Source: CAD feature listing. Evaluate the final solid. Frame: model axes, mm. A direction names the side the tool comes from. Give positions to 0.01 mm unless a question says otherwise; leave off trailing zeros. Write each loop counter-clockwise with the first axis right and the second up, starting at its lowest first coordinate (ties: lowest second). Pieces come first, ordered by that corner, then holes. Notation, with made-up numbers: (40, 62) -> (89, 62) arc R30 ccw to (89, 93) -> close; hole circle Ø5 at (-15.5, -2.5). An arc over 180 degrees is marked (long way). Write item = value, one per line.
from build123d import *

# Parameters (mm, degrees)
BOSS_EXTRUDE1_DEPTH     = 10
SKETCH3_W               = 5
SKETCH3_H               = 10
BOSS_EXTRUDE2_DEPTH     = 10
SKETCH5_R               = 2.5
CUT_EXTRUDE1_DEPTH      = 20
MIRROR2_COPY_1_SKETCH_W = 5
MIRROR2_COPY_1_SKETCH_H = 10
MIRROR2_COPY_1_DEPTH    = 10
MIRROR2_COPY_2_SKETCH_R = 2.5
MIRROR2_COPY_2_DEPTH    = 20


with BuildPart() as part:
    # Sketch1 → Boss-Extrude1 (new body)
    with BuildSketch(Plane(origin=(0, 0, 0), x_dir=(1, 0, 0), z_dir=(0, 1, 0))):
        Polygon((-381.1, 0), (-190.55, 330.042281382), (0, 0), align=None)
    extrude(amount=BOSS_EXTRUDE1_DEPTH)

    # Sketch3 → Boss-Extrude2 (add)
    with BuildSketch(Plane(origin=(0, 0, 0), x_dir=(-0.5, 0, -0.866025404), z_dir=(0.866025404, 0, -0.5))):
        with Locations((198.05, 5)):
            Rectangle(SKETCH3_W, SKETCH3_H)
        with Locations((183.05, 5)):
            Rectangle(SKETCH3_W, SKETCH3_H)
    boss_extrude2 = extrude(amount=BOSS_EXTRUDE2_DEPTH)

    # Sketch5 → Cut-Extrude1 (cut)
    with BuildSketch(Plane(origin=(-90.275, 0, -156.360886653), x_dir=(0.866025404, 0, -0.5), z_dir=(0.5, 0, 0.866025404))):
        with Locations((5, 5)):
            Circle(SKETCH5_R)
    cut_extrude1 = extrude(amount=-CUT_EXTRUDE1_DEPTH, mode=Mode.SUBTRACT)

    # Mirror1: Boss-Extrude2, Cut-Extrude1 across plane
    add(boss_extrude2.mirror(Plane(origin=(0, 0, 0), x_dir=(0.866025404, 0, 0.5), z_dir=(-0.5, 0, 0.866025404))))
    add(cut_extrude1.mirror(Plane(origin=(0, 0, 0), x_dir=(0.866025404, 0, 0.5), z_dir=(-0.5, 0, 0.866025404))), mode=Mode.SUBTRACT)

    # Mirror2: Boss-Extrude2, Cut-Extrude1 across plane
    add(boss_extrude2.mirror(Plane(origin=(-190.55, 0, 0), x_dir=(0, 0, 1), z_dir=(1, 0, 0))))
    add(cut_extrude1.mirror(Plane(origin=(-190.55, 0, 0), x_dir=(0, 0, 1), z_dir=(1, 0, 0))), mode=Mode.SUBTRACT)

    # Mirror2 copy 1 sketch → Mirror2 copy 1 (add)
    with BuildSketch(Plane(origin=(-381.1, 0, 0), x_dir=(1, 0, 0), z_dir=(0, 0, 1))):
        with Locations((198.05, 5)):
            Rectangle(MIRROR2_COPY_1_SKETCH_W, MIRROR2_COPY_1_SKETCH_H)
        with Locations((183.05, 5)):
            Rectangle(MIRROR2_COPY_1_SKETCH_W, MIRROR2_COPY_1_SKETCH_H)
    extrude(amount=MIRROR2_COPY_1_DEPTH)

    # Mirror2 copy 2 sketch → Mirror2 copy 2 (cut)
    with BuildSketch(Plane.ZY.offset(200.55)):
        with Locations((5, 5)):
            Circle(MIRROR2_COPY_2_SKETCH_R)
    extrude(amount=-MIRROR2_COPY_2_DEPTH, mode=Mode.SUBTRACT)


solid = part.part
1) Contact query for flat-ended pins moving along their axis: pin 1 (1.5 mm diameter, centred on x = -187, z = -152, fed in from -Y); pin 2 (4 mm diameter, centred on y = 7.5, z = -30.5, fed in from -X); pin 3 (1.5 mm diameter, centred on y = 1.5, z = -145.5, fed in from +X); pin 4 (5 mm diameter, centred on x = -312.5, y = 6, fed in from +Z). Output: stop coordinate, or through.
Computed:
pin_1 = 0
pin_2 = -364.65
pin_3 = -83.57
pin_4 = 0
2) Cut plane A-A (y = 5). State how many separate pieces and enclosed holes the cut face has, then the cut area to 3 significant figures.
Computed:
separate_pieces = 7
enclosed_holes = 0
area = 63,000 mm²
3) Access query for faces 1 (the flat face through (-87.93, 2.708, -157.715)), 2 (the flat face through (-180.55, 3, 3)), 3 (the flat face through (-290, 5, 0)). Directions: +Z, -Z, +X, -X, +Y, -Y. A direction counts if a zero-diameter tool reaches every point of the face in a straight line with its end or side. Return the directions, or none.
Computed:
face_1 = +X, +Y, -Y
face_2 = +Z, +X, +Y, -Y
face_3 = +Z, -X, +Y, -Y
4) Draft query along Z for faces 4 (the flat face through (-285.86, 4.93, -164.96)), 5 (the flat face through (-190, 5, 0)), 6 (the flat face through (-188, 0, -125)), 7 (the flat face through (-146.044, 4.93, -252.956)). Return one class per face: pulls with the +Z half, pulls with the -Z half, needs draft (parallel to the pull), parting line crosses it, or undercut.
Computed:
face_4 = undercut
face_5 = pulls with the +Z half
face_6 = needs draft
face_7 = pulls with the -Z half
5) Cut plane C-C (z = -272). Return the cut outline in (x, y), then the cut area to 3 significant figures.
Computed:
outline = (-224.06, 0) -> (-157.04, 0) -> (-157.04, 10) -> (-224.06, 10) -> close
area = 670 mm²
6) Material intervals for L1, parallel to Y at x = -181.6, z = 5; L2, parallel to Z at x = -209.5, y = 1.25; L3, parallel to Z at x = -182.15, y = 5, sorted ascending.
Computed:
L1 = 0 to 2.5, 7.5 to 10
L2 = -297.22 to 0
L3 = -315.49 to 2.5, 7.5 to 10
7) Cut plane B-B (x = -69). Return the cut outline in (y, z).
Computed:
outline = (0, -119.51) -> (10, -119.51) -> (10, 0) -> (0, 0) -> close
